Source: CAD feature listing. Evaluate the final solid. Frame: model axes, mm. Give positions to 0.01 mm unless a question says otherwise; leave off trailing zeros. Order: outer loops, then holes, each group sorted by start corner. A loop starts at its lowest first (then second) coordinate and runs counter-clockwise, first axis right, second up. Notation, with made-up numbers: M 57.25,-1 L 80.25,-1 A15 ccw 80.25,26 Z; hole C -18,10.5 d1. An arc over 180 degrees is marked long. Use CSV: the item, a comma, the result in double quotes. Start each with the question number.
Item 1: Pull-direction query (Z, two-part tool) for faces 1 (the face through (-47, -588, -14.294)), 2 (the face through (-69, -1192, 35)), 3 (the face through (-47, -588, -12.794)), 4 (the face through (-46, -588, 64.206)); classes: +Z half, -Z half, draft (parallel to the pull), parting line (faces both ways), or undercut.
Item 2: Ray query, probe 1 along X at (y, z) = (-592, 13.5); probe 2 along X at (y, z) = (-513.5, 60.5); probe 3 along Z at (x, y) = (-51, -854). Return the intervals inside material, ascending. Write a range as from..to.
Item 3: First-contact query: pin 1 (2 mm diameter, centred on y = -1040.5, z = 17, fed in from -X); pin 2 (6 mm diameter, centred on x = -28.5, z = 8.5, fed in from +Y); pin 3 (13 mm diameter, centred on y = -352.5, z = 25.5, fed in from +X); pin 4 (13 mm diameter, centred on y = -614, z = 26.5, fed in from -X). Flat tips, straight axial feed; report the tip coordinate or a pass-through.
Item 4: Section query A-A on x = -58.5. Return loops of the section in (y, z).
from build123d import *

# Parameters (mm, degrees)
F1_DEPTH = 1192
F2_T     = -1.5


with BuildPart() as f1:
    # F0 (on Front) → F1 (new body)
    with BuildSketch(Plane.XZ):
        with BuildLine():
            Line((-26.180391, 65.706456), (-66.371201, 65.706456))
            ThreePointArc((-66.371201, 65.706456), (-69.384465, 64.696474), (-71.180391, 62.074554))
            ThreePointArc((-71.180391, 62.074554), (-70.704452, 59.682332), (-69.349119, 57.654447))
            ThreePointArc((-69.349119, 57.654447), (-68.848906, 56.819509), (-68.802041, 55.847326))
            ThreePointArc((-68.802041, 55.847326), (-69.441389, 54.085616), (-70.574311, 52.592674))
            ThreePointArc((-70.574311, 52.592674), (-71.022651, 51.936965), (-71.180391, 51.158454))
            Line((-71.180391, 51.158454), (-71.180391, 37.170454))
            ThreePointArc((-71.180391, 37.170454), (-70.912442, 36.170454), (-70.180391, 35.438403))
            ThreePointArc((-70.180391, 35.438403), (-69.448341, 34.706352), (-69.180391, 33.706352))
            Line((-69.180391, 33.706352), (-69.180391, 17.706456))
            ThreePointArc((-69.180391, 17.706456), (-69.448341, 16.706456), (-70.180391, 15.974405))
            ThreePointArc((-70.180391, 15.974405), (-70.912442, 15.242355), (-71.180391, 14.242355))
            Line((-71.180391, 14.242355), (-71.180391, 1.642835))
            ThreePointArc((-71.180391, 1.642835), (-71.017419, 0.852057), (-70.555062, 0.190155))
            ThreePointArc((-70.555062, 0.190155), (-69.407243, -1.302963), (-68.778829, -3.078347))
            ThreePointArc((-68.778829, -3.078347), (-68.836672, -4.038251), (-69.335836, -4.860197))
            ThreePointArc((-69.335836, -4.860197), (-70.700856, -6.892661), (-71.180391, -9.293544))
            ThreePointArc((-71.180391, -9.293544), (-69.715925, -12.829078), (-66.180391, -14.293544))
            Line((-66.180391, -14.293544), (-26.371201, -14.293544))
            ThreePointArc((-26.371201, -14.293544), (-22.835667, -12.829078), (-21.371201, -9.293544))
            ThreePointArc((-21.371201, -9.293544), (-21.850737, -6.892661), (-23.215757, -4.860197))
            ThreePointArc((-23.215757, -4.860197), (-23.71492, -4.038251), (-23.772764, -3.078347))
            ThreePointArc((-23.772764, -3.078347), (-23.14435, -1.302963), (-21.99653, 0.190155))
            ThreePointArc((-21.99653, 0.190155), (-21.534174, 0.852057), (-21.371201, 1.642835))
            Line((-21.371201, 1.642835), (-21.371201, 14.242355))
            ThreePointArc((-21.371201, 14.242355), (-21.639151, 15.242355), (-22.371201, 15.974405))
            ThreePointArc((-22.371201, 15.974405), (-23.103252, 16.706456), (-23.371201, 17.706456))
            Line((-23.371201, 17.706456), (-23.371201, 33.706352))
            ThreePointArc((-23.371201, 33.706352), (-23.103252, 34.706352), (-22.371201, 35.438403))
            ThreePointArc((-22.371201, 35.438403), (-21.639151, 36.170454), (-21.371201, 37.170454))
            Line((-21.371201, 37.170454), (-21.371201, 51.158454))
            ThreePointArc((-21.371201, 51.158454), (-21.528942, 51.936965), (-21.977282, 52.592674))
            ThreePointArc((-21.977282, 52.592674), (-23.110203, 54.085616), (-23.749551, 55.847326))
            ThreePointArc((-23.749551, 55.847326), (-23.702687, 56.819509), (-23.202474, 57.654447))
            ThreePointArc((-23.202474, 57.654447), (-21.847141, 59.682332), (-21.371201, 62.074554))
            ThreePointArc((-21.371201, 62.074554), (-23.167128, 64.696474), (-26.180391, 65.706456))
        make_face()
    extrude(amount=F1_DEPTH)

    # F2
    f2_openings = [f1.faces().sort_by_distance(p)[0] for p in [
        (-46.275796, -1192, 25.7149),
        (-46.275796, 0, 25.7149),
    ]]
    offset(amount=F2_T, openings=f2_openings)


solid = f1.part
Verdict:
1,face 1,"-Z half"
1,face 2,"draft"
1,face 3,"undercut"
1,face 4,"undercut"
2,probe 1,"-71.18..-69.68, -22.87..-21.37"
2,probe 2,"-70.98..-69.41, -23.14..-21.57"
2,probe 3,"-14.29..-12.79, 64.21..65.71"
3,pin 1,"x = -70.14"
3,pin 2,"through"
3,pin 3,"x = -23.37"
3,pin 4,"x = -69.18"
4,outline,"M -1192,-14.29 L 0,-14.29 L 0,-12.79 L -1192,-12.79 Z; M -1192,64.21 L 0,64.21 L 0,65.71 L -1192,65.71 Z"
